Build history of the part. All positions in model axes, mm. Give positions to 0.01 mm unless a question says otherwise; leave off trailing zeros. Order: outer loops, then holes, each group sorted by start corner. A loop starts at its lowest first (then second) coordinate and runs counter-clockwise, first axis right, second up. Notation, with made-up numbers: (-39, 31.5) -> (-31, 31.5) arc R31 ccw to (-31, 58.5) -> close; hole circle Ø2 at (-20, 55). An arc over 180 degrees is marked (long way). One line per item, written item: value. Start each with the question number.
(1) Saw through at A-A on z = 0. Give the cut face in (x, y).
(2) Saw through at B-B on y = -14.25. Give the cut face in (x, z), plus the area to 3 significant figures.
(3) Probe line 1 (X direction, y = -6, z = -5); line 2 (X direction, y = -11, z = -9); line 3 (Z direction, x = 27, y = -22). List the from-to ranges inside material, lowest first.
(4) Two-plate mould, pull along Z, no slides. Class faces 1 (the cylindrical face through (59.173, -12.593, -0.552)), 2 (the cylindrical face through (2.982, -23.872, -23.643)), 3 (the cylindrical face through (23.995, -12.878, -7.739)): +Z half, -Z half, draft (parallel to the pull), parting line (faces both ways), or undercut.
(5) Saw through at C-C on x = -18. Give the cut face in (y, z), plus the area to 3 significant figures.
(6) Saw through at D-D on y = -2.25. Give the cut face in (x, z).
(7) Pin check, flat tips, straight feed: pin 1 (5 mm diameter, centred on y = -5, z = -5, fed in from +X); pin 2 (6 mm diameter, centred on y = -10, z = 10, fed in from +X); pin 3 (5 mm diameter, centred on y = -20.5, z = -10.5, fed in from +X). Stop position of each tip, or through.
```python
from build123d import *

# Parameters (mm, degrees)
F1_DEPTH = 25.4
F2_R     = 5.08
F3_R     = 12.717972
F4_DEPTH = 25.401


with BuildPart() as f1:
    # F0 (on Front) → F1 (new body)
    with BuildSketch(Plane.XZ):
        with BuildLine():
            ThreePointArc((34.087103, -25.091894), (59.178997, 0), (34.087103, 25.091894))
            Line((34.087103, 25.091894), (-34.087103, 25.091894))
            Line((-34.087103, 25.091894), (-34.087103, -25.091894))
            Line((-34.087103, -25.091894), (34.087103, -25.091894))
        make_face()
    extrude(amount=F1_DEPTH)

    # F2
    f2_edges = [f1.edges().sort_by_distance(p)[0] for p in [
        (0, -25.4, 25.091894),
        (-34.087103, -25.4, 0),
        (0, 0, -25.091894),
        (-34.087103, 0, 0),
        (-34.087103, -12.7, -25.091894),
        (-34.087103, -12.7, 25.091894),
    ]]
    fillet(f2_edges, radius=F2_R)

    # F3 (on face) → F4 (cut, through all)
    with BuildSketch(Plane.XZ.offset(25.4)):
        with Locations((34.087103, 0)):
            Circle(F3_R)
    extrude(amount=-F4_DEPTH, mode=Mode.SUBTRACT)


solid = f1.part
```
Results below:
1. outline: (-34.09, -20.32) arc R5.08 ccw to (-29.01, -25.4) -> (21.37, -25.4) -> (21.37, 0) -> (-29.01, 0) arc R5.08 ccw to (-34.09, -5.08) -> close; (46.81, -25.4) -> (54.1, -25.4) arc R5.08 ccw to (59.18, -20.32) -> (59.18, -5.08) arc R5.08 ccw to (54.1, 0) -> (46.81, 0) -> close
2. outline: (-34.09, -20.01) arc R5.08 ccw to (-29.01, -25.09) -> (34.09, -25.09) arc R25.09 ccw to (34.09, 25.09) -> (-29.01, 25.09) arc R5.08 ccw to (-34.09, 20.01) -> close; hole circle Ø25.44 at (34.09, 0)
2. area: 3,890 mm²
3. line 1: x = -34.09 to 22.39, 45.78 to 58.68
3. line 2: x = -34.09 to 25.1, 43.07 to 57.51
3. line 3: z = -24.81 to -10.56, 10.56 to 24.81
4. face 1: parting line
4. face 2: -Z half
4. face 3: undercut
5. outline: (-25.4, -20.01) arc R5.08 ccw to (-20.32, -25.09) -> (-5.08, -25.09) arc R5.08 ccw to (0, -20.01) -> (0, 20.01) arc R5.08 ccw to (-5.08, 25.09) -> (-20.32, 25.09) arc R5.08 ccw to (-25.4, 20.01) -> close
5. area: 1,250 mm²
6. outline: (-33.23, -20.01) arc R4.22 ccw to (-29.01, -24.23) -> (34.09, -24.23) arc R24.23 ccw to (34.09, 24.23) -> (-29.01, 24.23) arc R4.22 ccw to (-33.23, 20.01) -> close; hole circle Ø25.44 at (34.09, 0)
7. pin 1: stops at x = 59.05
7. pin 2: stops at x = 58.18
7. pin 3: stops at x = 57.87
